from build123d import *

# Parameters (mm, degrees)
SKETCH1_W           = 55
SKETCH1_H           = 34
BOSS_EXTRUDE1_DEPTH = 1.5
SKETCH3_R           = 1.125
CUT_EXTRUDE5_DEPTH  = 33.365104665


with BuildPart() as part:
    # Sketch1 → Boss-Extrude1 (new body)
    with BuildSketch(Plane(origin=(0, 0, 0), x_dir=(1, 0, 0), z_dir=(0, 1, 0))):
        Rectangle(SKETCH1_W, SKETCH1_H)
    extrude(amount=BOSS_EXTRUDE1_DEPTH)

    # Sketch3 → Cut-Extrude5 (cut, through all)
    with BuildSketch(Plane(origin=(0, 0, 0), x_dir=(1, 0, 0), z_dir=(0, 1, 0))):
        with Locations(Location((-18, 14.5, 0), (0, 0, 270))):
            Circle(SKETCH3_R)
        with Locations(Location((18, 14.5, 0), (0, 0, 270))):
            Circle(SKETCH3_R)
        with Locations(Location((-18, -14.5, 0), (0, 0, 270))):
            Circle(SKETCH3_R)
        with Locations(Location((18, -14.5, 0), (0, 0, 270))):
            Circle(SKETCH3_R)
        with Locations(Location((-25, 14.5, 0), (0, 0, 270))):
            Circle(SKETCH3_R)
        with Locations(Location((25, 14.5, 0), (0, 0, 270))):
            Circle(SKETCH3_R)
        with Locations(Location((25, -14.5, 0), (0, 0, 270))):
            Circle(SKETCH3_R)
        with Locations(Location((-25, -14.5, 0), (0, 0, 270))):
            Circle(SKETCH3_R)
    extrude(amount=CUT_EXTRUDE5_DEPTH, mode=Mode.SUBTRACT)


solid = part.part
The listing builds one solid part. Answer for the finished solid, in the listing's coordinates (mm). Coordinates: 2 decimals unless noted, no trailing zeros. Loops run counter-clockwise (first coordinate to the right, second up) from the corner with the lowest first, then second, coordinate; pieces in that order, holes last.
1) Determine the mould class of faces 1 (the face through (-27.5, 1, 0)), 2 (the face through (-17.05, 0.74, 15.1)), 3 (the face through (0, 1.5, 0)) for opening direction X: pulls with the +X half, pulls with the -X half, needs draft (parallel to the pull), parting line crosses it, or undercut.
2) Find section A-A on z = -14.5. Write down the section's boundary in (x, y) (3 decimals).
3) Find the intervals of material crossed by L1, parallel to Z at x = 18, y = 0.45 (3 decimals); L2, parallel to X at y = 0.45, z = -14.5 (3 decimals); L3, parallel to X at y = 0.65, z = -14, in increasing order.
4) Find section B-B on x = -18. Write down the section's boundary in (y, z) (3 decimals).
5) Find section C-C on y = 0.4. Give the number of separate pieces and of enclosed holes in the cut face, then the cut area to 3 significant figures.
Values:
1. face 1: pulls with the -X half
1. face 2: undercut
1. face 3: needs draft
2. outline: (-27.5, 0) - (-26.125, 0) - (-26.125, 1.5) - (-27.5, 1.5) - close; (-23.875, 0) - (-19.125, 0) - (-19.125, 1.5) - (-23.875, 1.5) - close; (-16.875, 0) - (16.875, 0) - (16.875, 1.5) - (-16.875, 1.5) - close; (19.125, 0) - (23.875, 0) - (23.875, 1.5) - (19.125, 1.5) - close; (26.125, 0) - (27.5, 0) - (27.5, 1.5) - (26.125, 1.5) - close
3. L1: z = -17 to -15.625, -13.375 to 13.375, 15.625 to 17
3. L2: x = -27.5 to -26.125, -23.875 to -19.125, -16.875 to 16.875, 19.125 to 23.875, 26.125 to 27.5
3. L3: x = -27.5 to -26.01, -23.99 to -19.01, -16.99 to 16.99, 19.01 to 23.99, 26.01 to 27.5
4. outline: (0, -17) - (1.5, -17) - (1.5, -15.625) - (0, -15.625) - close; (0, -13.375) - (1.5, -13.375) - (1.5, 13.375) - (0, 13.375) - close; (0, 15.625) - (1.5, 15.625) - (1.5, 17) - (0, 17) - close
5. separate pieces: 1
5. enclosed holes: 8
5. area: 1,840 mm2
